Geometry check sheet. Reference: drawing and pictorial views, mm from the part's lowest x, y, z. Give positions to 0.01 mm unless a question says otherwise; leave off trailing zeros. Loops run counter-clockwise (first coordinate to the right, second up) from the corner with the lowest first, then second, coordinate; pieces in that order, holes last. Notation, with made-up numbers: (62.25, -36) -> (85.25, -36) arc R32 cw to (85.25, -8) -> close; hole circle Ø4 at (2.25, -2.75). An arc over 180 degrees is marked (long way). Write each question's results on one line, items separated by ' | '. Start each with the question number.
1. Material ranges on L1, parallel to Y at x = 120, z = 3.95; L2, parallel to X at y = 130, z = 1.15; L3, parallel to Y at x = 20, z = 1.3, recorded low to high. Write a range as from..to.
2. Cross-section at D-D on x = 20. Record the boundary of the cut face in (y, z), and give its area (3 significant figures).
3. Cross-section at A-A on x = 120. Record the boundary of the cut face in (y, z), and give its area (3 significant figures).
4. Cross-section at C-C on z = 1.6. Count the separate pieces of the cut face and the enclosed holes in it, and give its area (3 significant figures).
5. Cross-section at B-B on y = 73. Record the boundary of the cut face in (x, z).
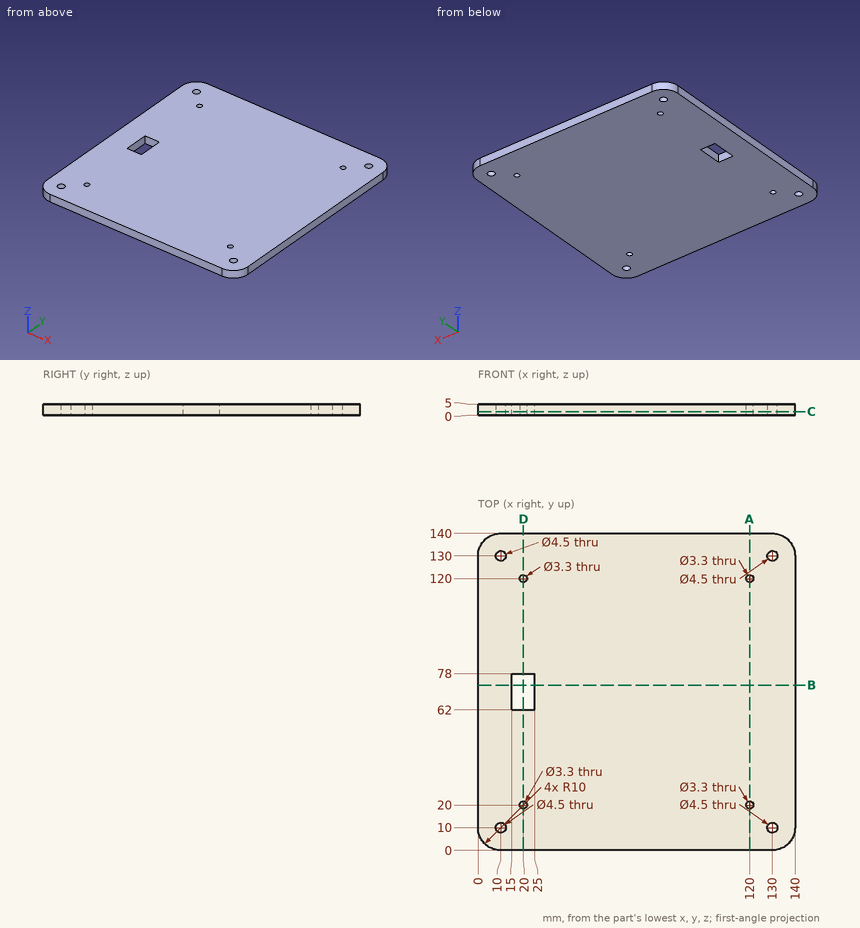
Geometry says:
1) L1: 0..18.35, 21.65..118.35, 121.65..140 | L2: 0..7.75, 12.25..127.75, 132.25..140 | L3: 0..18.35, 21.65..62, 78..118.35, 121.65..140
2) outline: (0, 0) -> (18.35, 0) -> (18.35, 5) -> (0, 5) -> close; (21.65, 0) -> (62, 0) -> (62, 5) -> (21.65, 5) -> close; (78, 0) -> (118.35, 0) -> (118.35, 5) -> (78, 5) -> close; (121.65, 0) -> (140, 0) -> (140, 5) -> (121.65, 5) -> close | area: 587 mm^2
3) outline: (0, 0) -> (18.35, 0) -> (18.35, 5) -> (0, 5) -> close; (21.65, 0) -> (118.35, 0) -> (118.35, 5) -> (21.65, 5) -> close; (121.65, 0) -> (140, 0) -> (140, 5) -> (121.65, 5) -> close | area: 667 mm^2
4) separate pieces: 1 | enclosed holes: 9 | area: 19,300 mm^2
5) outline: (0, 0) -> (15, 0) -> (15, 5) -> (0, 5) -> close; (25, 0) -> (140, 0) -> (140, 5) -> (25, 5) -> close
